Verification items for the finished model (mm, model axes). Face numbers are marked on the shaded views. A direction names the side the tool comes from. Give positions to 0.01 mm unless a question says otherwise; leave off trailing zeros. Write each loop counter-clockwise with the first axis right and the second up, starting at its lowest first coordinate (ties: lowest second). Pieces come first, ordered by that corner, then holes. Notation, with made-up numbers: (32.5, 21) -> (50.5, 21) arc R21 cw to (50.5, 34) -> close; hole circle Ø1 at (51, -27.75). An arc over 180 degrees is marked (long way). Write item = value, one per line.
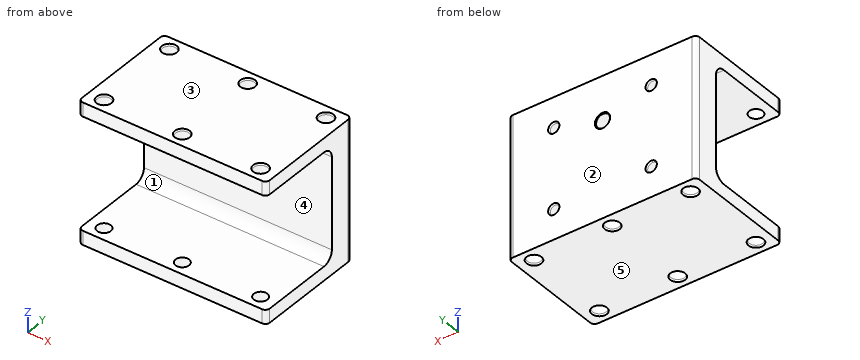
from build123d import *

# Parameters (mm, degrees)
SKETCH1_W             = 108
SKETCH1_H             = 80.5
BOSS_EXTRUDE1_DEPTH   = 15
SKETCH2_R             = 3.9
CUT_EXTRUDE1_DEPTH    = 7
SKETCH3_W             = 108
SKETCH3_H             = 50
SKETCH3_R             = 3.9
BOSS_EXTRUDE2_DEPTH   = 8
CHAMFER1_SIZE         = 0.4
CHAMFER1_SIZE2        = 1.098990968
CHAMFER1_PART_2_SIZE  = 0.4
CHAMFER1_PART_2_SIZE2 = 1.098990968
FILLET1_R             = 2.5
FILLET2_R             = 6
SKETCH4_R             = 2.85
CUT_EXTRUDE2_DEPTH    = 11
CHAMFER2_SIZE         = 0.4
CHAMFER2_SIZE2        = 1.098990968
SKETCH5_R             = 4
CUT_EXTRUDE3_DEPTH    = 66
CHAMFER3_SIZE         = 0.4


with BuildPart() as part:
    # Sketch1 → Boss-Extrude1 (new body)
    with BuildSketch(Plane(origin=(0, 0, 0), x_dir=(1, 0, 0), z_dir=(0, 1, 0))):
        with Locations((54, 40.25)):
            Rectangle(SKETCH1_W, SKETCH1_H)
    extrude(amount=BOSS_EXTRUDE1_DEPTH)

    # Sketch2 → Cut-Extrude1 (cut)
    with BuildSketch(Plane.XY):
        with Locations((9, 7.5)):
            Circle(SKETCH2_R)
        with Locations((99, 7.5)):
            Circle(SKETCH2_R)
        with Locations((54, 7.5)):
            Circle(SKETCH2_R)
    cut_extrude1 = extrude(amount=-CUT_EXTRUDE1_DEPTH, mode=Mode.SUBTRACT)

    # Sketch3 → Boss-Extrude2 (add)
    with BuildSketch(Plane.XY):
        with Locations((54, -25)):
            Rectangle(SKETCH3_W, SKETCH3_H)
        with Locations((99, -42.5)):
            Circle(SKETCH3_R, mode=Mode.SUBTRACT)
        with Locations((54, -42.5)):
            Circle(SKETCH3_R, mode=Mode.SUBTRACT)
        with Locations((9, -42.5)):
            Circle(SKETCH3_R, mode=Mode.SUBTRACT)
    boss_extrude2 = extrude(amount=-BOSS_EXTRUDE2_DEPTH)

    # Mirror1: Cut-Extrude1, Boss-Extrude2 across plane
    add(cut_extrude1.mirror(Plane.XY.offset(-40.25)), mode=Mode.SUBTRACT)
    add(boss_extrude2.mirror(Plane.XY.offset(-40.25)))

    # Chamfer1
    chamfer1_edges = [part.edges().sort_by_distance(p)[0] for p in [
        (5.1, 7.5, 0),
        (95.1, 7.5, 0),
        (50.1, 7.5, 0),
        (95.1, -42.5, 0),
        (50.1, -42.5, 0),
        (5.1, -42.5, 0),
    ]]
    chamfer1_side = [part.faces().sort_by_distance(p)[0] for p in [
        (54, -17.5, 0),
    ]]
    chamfer(chamfer1_edges, length=CHAMFER1_SIZE, length2=CHAMFER1_SIZE2, reference=chamfer1_side[0])

    # Chamfer1 part 2
    chamfer1_part_2_edges = [part.edges().sort_by_distance(p)[0] for p in [
        (5.1, 7.5, -80.5),
        (95.1, 7.5, -80.5),
        (50.1, 7.5, -80.5),
        (50.1, -42.5, -80.5),
        (95.1, -42.5, -80.5),
        (5.1, -42.5, -80.5),
    ]]
    chamfer1_part_2_side = [part.faces().sort_by_distance(p)[0] for p in [
        (54, -17.5, -80.5),
    ]]
    chamfer(chamfer1_part_2_edges, length=CHAMFER1_PART_2_SIZE, length2=CHAMFER1_PART_2_SIZE2, reference=chamfer1_part_2_side[0])

    # Fillet1
    fillet1_edges = [part.edges().sort_by_distance(p)[0] for p in [
        (108, 15, -40.25),
        (0, -50, -4),
        (108, -50, -4),
        (0, 15, -40.25),
        (0, -50, -76.5),
        (108, -50, -76.5),
    ]]
    fillet(fillet1_edges, radius=FILLET1_R)

    # Fillet2
    fillet2_edges = [part.edges().sort_by_distance(p)[0] for p in [
        (54, 0, -8),
        (54, 0, -72.5),
    ]]
    fillet(fillet2_edges, radius=FILLET2_R)

    # Sketch4 → Cut-Extrude2 (cut)
    with BuildSketch(Plane(origin=(0, 15, 0), x_dir=(1, 0, 0), z_dir=(0, 1, 0))):
        with Locations((82, 17.25)):
            Circle(SKETCH4_R)
        with Locations((26, 17.25)):
            Circle(SKETCH4_R)
        with Locations((26, 63.25)):
            Circle(SKETCH4_R)
        with Locations((82, 63.25)):
            Circle(SKETCH4_R)
    extrude(amount=-CUT_EXTRUDE2_DEPTH, mode=Mode.SUBTRACT)

    # Chamfer2
    chamfer2_edges = [part.edges().sort_by_distance(p)[0] for p in [
        (79.15, 15, -63.25),
        (23.15, 15, -63.25),
        (23.15, 15, -17.25),
        (79.15, 15, -17.25),
    ]]
    chamfer2_side = [part.faces().sort_by_distance(p)[0] for p in [
        (54, 15, -40.25),
    ]]
    chamfer(chamfer2_edges, length=CHAMFER2_SIZE, length2=CHAMFER2_SIZE2, reference=chamfer2_side[0])

    # Sketch5 → Cut-Extrude3 (cut, through all)
    with BuildSketch(Plane(origin=(0, 15, 0), x_dir=(1, 0, 0), z_dir=(0, 1, 0))):
        with Locations((54, 25.25)):
            Circle(SKETCH5_R)
    extrude(amount=-CUT_EXTRUDE3_DEPTH, mode=Mode.SUBTRACT)

    # Chamfer3
    chamfer3_edges = [part.edges().sort_by_distance(p)[0] for p in [
        (50, 15, -25.25),
    ]]
    chamfer(chamfer3_edges, length=CHAMFER3_SIZE)


solid = part.part
Item 1: Mould release check, pull along Z, two halves, no side actions. Record for the marked faces 1, 2 and 3: +Z half, -Z half, draft (parallel to the pull), parting line (faces both ways), or undercut.
Response values:
face_1 = undercut
face_2 = draft
face_3 = +Z half
Item 2: Sectioned sample at B-B on x = 9. Give the number of separate pieces and of enclosed holes in the cut face, then the cut area to 3 significant figures.
Response values:
separate_pieces = 3
enclosed_holes = 0
area = 1,790 mm^2
Item 3: Sectioned sample at D-D on x = 82. Record the cut outline in (y, z).
Response values:
outline = (-50, -80.5) -> (15, -80.5) -> (15, -66.5) -> (13.9, -66.1) -> (4, -66.1) -> (4, -60.4) -> (13.9, -60.4) -> (15, -60) -> (15, -20.5) -> (13.9, -20.1) -> (4, -20.1) -> (4, -14.4) -> (13.9, -14.4) -> (15, -14) -> (15, 0) -> (-50, 0) -> (-50, -8) -> (-6, -8) arc R6 cw to (0, -14) -> (0, -66.5) arc R6 cw to (-6, -72.5) -> (-50, -72.5) -> close
Item 4: Sectioned sample at A-A on y = -35. Record the cut outline in (x, z).
Response values:
outline = (0, -80.5) -> (108, -80.5) -> (108, -72.5) -> (0, -72.5) -> close; (0, -8) -> (108, -8) -> (108, 0) -> (0, 0) -> close
Item 5: Material ranges on line 1 (Y direction, x = 99, z = -77.8); line 2 (X direction, y = 10.5, z = -63.25); line 3 (Z direction, x = 88, y = -20.5), recorded low to high.
Response values:
line_1 = -50 to -46.4, -38.6 to 3.6, 11.4 to 15
line_2 = 0 to 23.15, 28.85 to 79.15, 84.85 to 108
line_3 = -80.5 to -72.5, -8 to 0
Item 6: Set-up check for the marked faces 4 and 5: record each of +Z, -Z, +X, -X, +Y, -Y from which the full face is reachable in a straight line by a thin tool's end or side.
Response values:
face_4 = +X, -X, -Y
face_5 = -Z, +X, -X, +Y, -Y
Item 7: Go/stop test with flat-tipped pins: P1, Ø4, axis at x = 44.5, y = -21.5, coming from the +Z side; P2, Ø4, axis at x = 10.5, y = 6.5, coming from the -Z side; P3, Ø6, axis at x = 54, y = 7.5, coming from the +Z side. Record where each tip stops, or that it passes through.
Response values:
P1 = 0
P2 = -73.5
P3 = -7
Item 8: Sectioned sample at C-C on z = -25.25. Record the cut outline in (x, y), then the cut area to 3 significant figures.
Response values:
outline = (0, 0) -> (50, 0) -> (50, 14.6) -> (49.6, 15) -> (2.5, 15) arc R2.5 ccw to (0, 12.5) -> close; (58, 0) -> (108, 0) -> (108, 12.5) arc R2.5 ccw to (105.5, 15) -> (58.4, 15) -> (58, 14.6) -> close
area = 1,500 mm^2
